```python
from build123d import *

# Parameters (mm, degrees)
SKETCH2_R = 1.29413


with BuildPart() as part:
    # Sweep1: sweep along a path in Sketch1
    with BuildLine(Plane(origin=(0, 0, 0), x_dir=(1, 0, 0), z_dir=(0, 1, 0))) as sweep1_path:
        Line((0, 2.58826), (120, 2.58826))
        ThreePointArc((120, 2.58826), (128.880770004, -0.4263552), (134.091177095, -8.224280477))
        Line((134.091177095, -8.224280477), (134.895024672, -11.224280477))
        ThreePointArc((134.895024672, -11.224280477), (135.267302991, -13.095849971), (135.392107577, -15))
        Line((135.392107577, -15), (135.392107577, -26))
    # Sketch2 → Sweep1 (sweep)
    with BuildSketch(Plane(origin=(0, 0, 0), x_dir=(0, 0, -1), z_dir=(1, 0, 0))):
        with Locations((2.58826, 0)):
            Circle(SKETCH2_R)
    sweep1 = sweep(path=sweep1_path.line)

    # Mirror1: Sweep1 across plane
    add(sweep1.mirror(Plane(origin=(0, 0, 0), x_dir=(0, 0, 1), z_dir=(1, 0, 0))))


solid = part.part
```
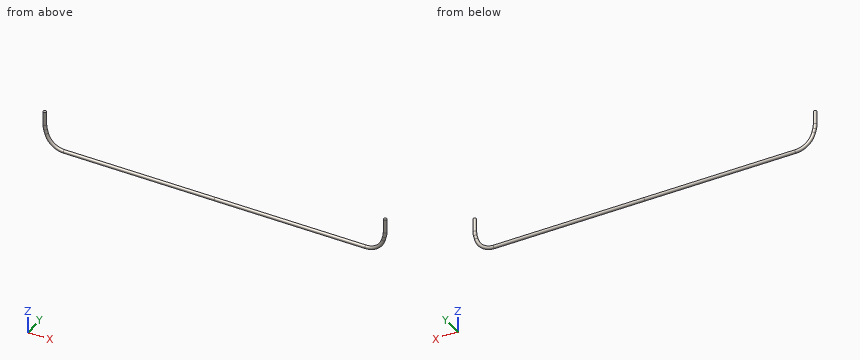
Input: part model. Units: mm. Frame: model coordinates. Give positions to 0.01 mm unless a question says otherwise; leave off trailing zeros. Order: outer loops, then holes, each group sorted by start corner. A loop starts at its lowest first (then second) coordinate and runs counter-clockwise, first axis right, second up.
1. Section A-A on y = 0. Return the cut outline in (x, z) (3 decimals).
Derived:
outline: (-136.686, 15) arc R15.882 ccw to (-136.145, 10.889) - (-135.341, 7.889) arc R15.882 ccw to (-120, -3.882) - (120, -3.882) arc R15.882 ccw to (135.341, 7.889) - (136.145, 10.889) arc R15.882 ccw to (136.686, 15) - (136.686, 26) - (134.098, 26) - (134.098, 15) arc R13.294 cw to (133.645, 11.559) - (132.841, 8.559) arc R13.294 cw to (120, -1.294) - (-120, -1.294) arc R13.294 cw to (-132.841, 8.559) - (-133.645, 11.559) arc R13.294 cw to (-134.098, 15) - (-134.098, 26) - (-136.686, 26) - close
2. Section C-C on x = -94. Return the cut outline in (y, z).
Derived:
outline: circle Ø2.59 at (0, -2.59)
3. Pin query (flat end, axial travel): pin 1 (1.5 mm diameter, centred on x = 95, y = -1, fed in from +Z). Return the tip coordinate at first contact, or that it passes through.
Derived:
pin 1: stops at z = -1.32
4. Material intervals for L1, parallel to X at y = 0.05, z = 18.25; L2, parallel to Z at x = 81, y = 0.15; L3, parallel to X at y = 0.4, z = 6.5, sorted ascending.
Derived:
L1: x = -136.69 to -134.1, 134.1 to 136.69
L2: z = -3.87 to -1.3
L3: x = -134.83 to -132.17, 132.17 to 134.83
5. Section B-B on z = 18.5. Return the cut outline in (x, y).
Derived:
outline: circle Ø2.59 at (-135.39, 0); circle Ø2.59 at (135.39, 0)
